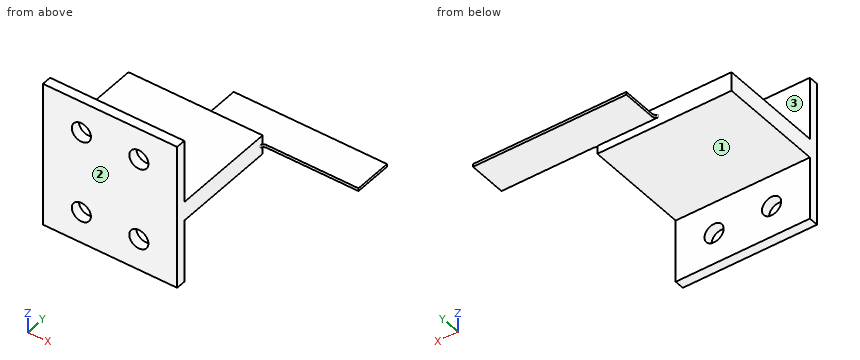
from build123d import *

# Parameters (mm, degrees)
ESQUISSE1_W             = 35
ESQUISSE1_H             = 5
BOSS_EXTRU_1_DEPTH      = 30
ESQUISSE2_W             = 40
ESQUISSE2_H             = 0.75
BOSS_EXTRU_2_DEPTH      = 10
CONG_1_R                = 1
ESQUISSE3_W             = 35
ESQUISSE3_H             = 38.1
BOSS_EXTRU_3_DEPTH      = 2.5
ESQUISSE4_R             = 2.5
ENL_V_MAT_EXTRU_1_DEPTH = 2.5


with BuildPart() as part:
    # Esquisse1 → Boss.-Extru.1 (new body)
    with BuildSketch(Plane(origin=(0, 0, 0), x_dir=(1, 0, 0), z_dir=(0, 1, 0))):
        Rectangle(ESQUISSE1_W, ESQUISSE1_H)
    extrude(amount=BOSS_EXTRU_1_DEPTH)

    # Esquisse2 → Boss.-Extru.2 (add)
    with BuildSketch(Plane(origin=(0, 30, 0), x_dir=(1, 0, 0), z_dir=(0, 1, 0))):
        with Locations((22.5, 0)):
            Rectangle(ESQUISSE2_W, ESQUISSE2_H)
    extrude(amount=BOSS_EXTRU_2_DEPTH)

    # Congé1
    cong_1_edges = [part.edges().sort_by_distance(p)[0] for p in [
        (17.5, 30, 0),
        (2.5, 30, 0),
    ]]
    fillet(cong_1_edges, radius=CONG_1_R)

    # Esquisse3 → Boss.-Extru.3 (add)
    with BuildSketch(Plane.XZ):
        Rectangle(ESQUISSE3_W, ESQUISSE3_H)
    extrude(amount=-BOSS_EXTRU_3_DEPTH)

    # Esquisse4 → Enlèv. mat.-Extru.1 (cut)
    with BuildSketch(Plane(origin=(0, 2.5, 0), x_dir=(1, 0, 0), z_dir=(0, 1, 0))):
        with Locations((-7.5, 10.775)):
            Circle(ESQUISSE4_R)
        with Locations((7.5, 10.775)):
            Circle(ESQUISSE4_R)
        with Locations((7.5, -10.775)):
            Circle(ESQUISSE4_R)
        with Locations((-7.5, -10.775)):
            Circle(ESQUISSE4_R)
    extrude(amount=-ENL_V_MAT_EXTRU_1_DEPTH, mode=Mode.SUBTRACT)


solid = part.part
Verification items for the finished model (mm, model axes). Face numbers are marked on the shaded views. A direction names the side the tool comes from. Coordinates: 2 decimals unless noted, no trailing zeros. Order: outer loops, then holes, each group sorted by start corner. A loop starts at its lowest first (then second) coordinate and runs counter-clockwise, first axis right, second up. Notation, with made-up numbers: (53, -8) -> (83, -8) arc R25 cw to (83, 29) -> close; hole circle Ø11 at (-8.75, -32). An arc over 180 degrees is marked (long way). Use CSV: the item, a comma, the result in double quotes. Start each with the question number.
Q1. Section check D-D, the plane z = 6.5. Record the cut outline in (x, y), and give its area (3 significant figures).
Q2. Section check C-C, the plane x = -7.5. Record the cut outline in (y, z) (3 decimals), and give its area (3 significant figures).
Q3. Tool access check on the marked faces 1, 2 and 3. Record the directions out of +Z, -Z, +X, -X, +Y, -Y that give a thin tool (end or side, any length) a straight path to the whole face; none if there is none.
Q4. Section check A-A, the plane x = 7.5. Record the cut outline in (y, z) (3 decimals), and give its area (3 significant figures).
Q5. Thickness scan on line 1 along Z through (x, y) = (7.5, 1.7) (3 decimals); line 2 along Y through (x, z) = (-12, 11); line 3 along Z through (x, y) = (27, 30.5) (3 decimals). Record the ranges inside material, lowest first.
Q6. Depth check by flat-ended pin: P1, Ø3, axis at y = 6.5, z = -3.5, coming from the +X side; P2, Ø4, axis at x = 33, y = 34.5, coming from the +Z side (3 decimals); P3, Ø6, axis at x = -1.5, y = 26.5, coming from the -Z side. Enter the tip coordinate at first touch or a pass-through.
Q7. Section check B-B, the plane x = -0.5. Record the cut outline in (y, z), and give its area (3 significant figures).
Returned:
1,outline,"(-17.5, 0) -> (17.5, 0) -> (17.5, 2.5) -> (-17.5, 2.5) -> close"
1,area,"87.5 mm^2"
2,outline,"(0, -19.05) -> (2.5, -19.05) -> (2.5, -13.275) -> (0, -13.275) -> close; (0, -8.275) -> (2.5, -8.275) -> (2.5, -2.5) -> (30, -2.5) -> (30, 2.5) -> (2.5, 2.5) -> (2.5, 8.275) -> (0, 8.275) -> close; (0, 13.275) -> (2.5, 13.275) -> (2.5, 19.05) -> (0, 19.05) -> close"
2,area,"208 mm^2"
3,face 1,"-Z, +X, -X, +Y"
3,face 2,"+Z, -Z, +X, -X, -Y"
3,face 3,"+Z, +X, -X, +Y"
4,outline,"(0, -19.05) -> (2.5, -19.05) -> (2.5, -13.275) -> (0, -13.275) -> close; (0, -8.275) -> (2.5, -8.275) -> (2.5, -2.5) -> (30, -2.5) -> (30, -0.375) -> (40, -0.375) -> (40, 0.375) -> (30, 0.375) -> (30, 2.5) -> (2.5, 2.5) -> (2.5, 8.275) -> (0, 8.275) -> close; (0, 13.275) -> (2.5, 13.275) -> (2.5, 19.05) -> (0, 19.05) -> close"
4,area,"215 mm^2"
5,line 1,"z = -19.05 to -13.275, -8.275 to 8.275, 13.275 to 19.05"
5,line 2,"y = 0 to 2.5"
5,line 3,"z = -0.375 to 0.375"
6,P1,"stops at x = 17.5"
6,P2,"stops at z = 0.375"
6,P3,"stops at z = -2.5"
7,outline,"(0, -19.05) -> (2.5, -19.05) -> (2.5, -2.5) -> (30, -2.5) -> (30, 2.5) -> (2.5, 2.5) -> (2.5, 19.05) -> (0, 19.05) -> close"
7,area,"233 mm^2"
